```python
from build123d import *

# Parameters (mm, degrees)
F0_W     = 4
F0_H     = 1
F1_DEPTH = 1
F2_DEPTH = 6
F3_DEPTH = 2
F3_TAPER = -1


with BuildPart() as f1:
    # F0 (on Top) → F1 (new body)
    with BuildSketch(Plane.XY):
        with BuildLine():
            Line((-13, 24.5), (-12, 24.5))
            Line((-12, 24.5), (-10.5, 24.5))
            Line((-10.5, 24.5), (-8, 24.5))
            Line((-8, 24.5), (-8, 25.5))
            Line((-8, 25.5), (-8, 26.5))
            Line((-8, 26.5), (-14, 26.5))
            ThreePointArc((-14, 26.5), (-14.7071067812, 26.2071067812), (-15, 25.5))
            Line((-15, 25.5), (-15, -25.5))
            ThreePointArc((-15, -25.5), (-14.7071067812, -26.2071067812), (-14, -26.5))
            Line((-14, -26.5), (14, -26.5))
            ThreePointArc((14, -26.5), (14.7071067812, -26.2071067812), (15, -25.5))
            Line((15, -25.5), (15, 25.5))
            ThreePointArc((15, 25.5), (14.7071067812, 26.2071067812), (14, 26.5))
            Line((14, 26.5), (8, 26.5))
            Line((8, 26.5), (8, 25.5))
            Line((8, 25.5), (8, 24.5))
            Line((8, 24.5), (10.5, 24.5))
            Line((10.5, 24.5), (12, 24.5))
            ThreePointArc((12, 24.5), (12.7071067812, 24.2071067812), (13, 23.5))
            Line((13, 23.5), (13, 22))
            Line((13, 22), (13, -22))
            Line((13, -22), (13, -23.5))
            ThreePointArc((13, -23.5), (12.7071067812, -24.2071067812), (12, -24.5))
            Line((12, -24.5), (10.5, -24.5))
            Line((10.5, -24.5), (-10.5, -24.5))
            Line((-10.5, -24.5), (-12, -24.5))
            ThreePointArc((-12, -24.5), (-12.7071067812, -24.2071067812), (-13, -23.5))
            Line((-13, -23.5), (-13, -22))
            Line((-13, -22), (-13, 22))
            Line((-13, 22), (-13, 23.5))
            Line((-13, 23.5), (-13, 24.5))
        make_face()
        with Locations((6, 25)):
            Rectangle(F0_W, F0_H)
        with Locations((2, 25)):
            Rectangle(F0_W, F0_H)
        with Locations((-2, 25)):
            Rectangle(F0_W, F0_H)
        with Locations((-6, 25)):
            Rectangle(F0_W, F0_H)
        Polygon((0, 24.5), (-4, 24.5), (-4, 20), (4, 20), (4, 24.5), align=None)
        with BuildLine():
            Line((-12, -22), (-13, -22))
            Line((-13, -22), (-13, -23.5))
            ThreePointArc((-13, -23.5), (-12.7071067812, -24.2071067812), (-12, -24.5))
            Line((-12, -24.5), (-10.5, -24.5))
            Line((-10.5, -24.5), (-10.5, -23.5))
            ThreePointArc((-10.5, -23.5), (-11.5606601718, -23.0606601718), (-12, -22))
        make_face()
        with BuildLine():
            Line((-8, 24.5), (-10.5, 24.5))
            Line((-10.5, 24.5), (-10.5, 23.5))
            ThreePointArc((-10.5, 23.5), (-9.4393398282, 23.0606601718), (-9, 22))
            ThreePointArc((-9, 22), (-10.5, 20.5), (-12, 22))
            Line((-12, 22), (-13, 22))
            Line((-13, 22), (-13, -22))
            Line((-13, -22), (-12, -22))
            ThreePointArc((-12, -22), (-10.5, -20.5), (-9, -22))
            ThreePointArc((-9, -22), (-9.4393398282, -23.0606601718), (-10.5, -23.5))
            Line((-10.5, -23.5), (-10.5, -24.5))
            Line((-10.5, -24.5), (10.5, -24.5))
            Line((10.5, -24.5), (10.5, -23.5))
            ThreePointArc((10.5, -23.5), (9.4393398282, -20.9393398282), (12, -22))
            Line((12, -22), (13, -22))
            Line((13, -22), (13, 22))
            Line((13, 22), (12, 22))
            ThreePointArc((12, 22), (9.4393398282, 20.9393398282), (10.5, 23.5))
            Line((10.5, 23.5), (10.5, 24.5))
            Line((10.5, 24.5), (8, 24.5))
            Line((8, 24.5), (4, 24.5))
            Line((4, 24.5), (4, 20))
            Line((4, 20), (-4, 20))
            Line((-4, 20), (-4, 24.5))
            Line((-4, 24.5), (-8, 24.5))
        make_face()
        with BuildLine():
            Line((10.5, -23.5), (10.5, -24.5))
            Line((10.5, -24.5), (12, -24.5))
            ThreePointArc((12, -24.5), (12.7071067812, -24.2071067812), (13, -23.5))
            Line((13, -23.5), (13, -22))
            Line((13, -22), (12, -22))
            ThreePointArc((12, -22), (11.5606601718, -23.0606601718), (10.5, -23.5))
        make_face()
        with BuildLine():
            Line((12, 24.5), (10.5, 24.5))
            Line((10.5, 24.5), (10.5, 23.5))
            ThreePointArc((10.5, 23.5), (11.5606601718, 23.0606601718), (12, 22))
            Line((12, 22), (13, 22))
            Line((13, 22), (13, 23.5))
            ThreePointArc((13, 23.5), (12.7071067812, 24.2071067812), (12, 24.5))
        make_face()
        with BuildLine():
            Line((-10.5, 24.5), (-12, 24.5))
            ThreePointArc((-12, 24.5), (-12.7071067812, 24.2071067812), (-13, 23.5))
            Line((-13, 23.5), (-13, 22))
            Line((-13, 22), (-12, 22))
            ThreePointArc((-12, 22), (-11.5606601718, 23.0606601718), (-10.5, 23.5))
            Line((-10.5, 23.5), (-10.5, 24.5))
        make_face()
        with BuildLine():
            ThreePointArc((-13, 23.5), (-12.7071067812, 24.2071067812), (-12, 24.5))
            Line((-12, 24.5), (-13, 24.5))
            Line((-13, 24.5), (-13, 23.5))
        make_face()
    extrude(amount=F1_DEPTH)

    # F0 (on Top) → F2 (join)
    with BuildSketch(Plane.XY):
        with BuildLine():
            Line((-13, 24.5), (-12, 24.5))
            Line((-12, 24.5), (-10.5, 24.5))
            Line((-10.5, 24.5), (-8, 24.5))
            Line((-8, 24.5), (-8, 25.5))
            Line((-8, 25.5), (-8, 26.5))
            Line((-8, 26.5), (-14, 26.5))
            ThreePointArc((-14, 26.5), (-14.7071067812, 26.2071067812), (-15, 25.5))
            Line((-15, 25.5), (-15, -25.5))
            ThreePointArc((-15, -25.5), (-14.7071067812, -26.2071067812), (-14, -26.5))
            Line((-14, -26.5), (14, -26.5))
            ThreePointArc((14, -26.5), (14.7071067812, -26.2071067812), (15, -25.5))
            Line((15, -25.5), (15, 25.5))
            ThreePointArc((15, 25.5), (14.7071067812, 26.2071067812), (14, 26.5))
            Line((14, 26.5), (8, 26.5))
            Line((8, 26.5), (8, 25.5))
            Line((8, 25.5), (8, 24.5))
            Line((8, 24.5), (10.5, 24.5))
            Line((10.5, 24.5), (12, 24.5))
            ThreePointArc((12, 24.5), (12.7071067812, 24.2071067812), (13, 23.5))
            Line((13, 23.5), (13, 22))
            Line((13, 22), (13, -22))
            Line((13, -22), (13, -23.5))
            ThreePointArc((13, -23.5), (12.7071067812, -24.2071067812), (12, -24.5))
            Line((12, -24.5), (10.5, -24.5))
            Line((10.5, -24.5), (-10.5, -24.5))
            Line((-10.5, -24.5), (-12, -24.5))
            ThreePointArc((-12, -24.5), (-12.7071067812, -24.2071067812), (-13, -23.5))
            Line((-13, -23.5), (-13, -22))
            Line((-13, -22), (-13, 22))
            Line((-13, 22), (-13, 23.5))
            Line((-13, 23.5), (-13, 24.5))
        make_face()
        with Locations((6, 25)):
            Rectangle(F0_W, F0_H)
        with Locations((-6, 25)):
            Rectangle(F0_W, F0_H)
    extrude(amount=F2_DEPTH)

    # F0 (on Top) → F3 (join)
    with BuildSketch(Plane.XY):
        Polygon((0, 24.5), (-4, 24.5), (-4, 20), (4, 20), (4, 24.5), align=None)
    extrude(amount=F3_DEPTH, taper=F3_TAPER)


solid = f1.part
```
The model under review builds one solid part; all positions refer to its coordinate system, in mm. A direction names the side the tool comes from. Coordinates: 2 decimals unless noted, no trailing zeros. Order: outer loops, then holes, each group sorted by start corner. A loop starts at its lowest first (then second) coordinate and runs counter-clockwise, first axis right, second up. Notation, with made-up numbers: M -1,-7 L 41,-7 A14 cw 41,17 Z; hole C 4.25,61.25 d4. An arc over 180 degrees is marked long. One line per question, with ' | ' between items.
(1) For probe 1 along Y at (x, z) = (10.5, 0.55); probe 2 along X at (y, z) = (-22, 0.2); probe 3 along Y at (x, z) = (10.5, 3.5), list the stretches that pass through material, from the lowest coordinate up. Write a range as from..to.
Geometry results:
probe 1: y = -26.5..-23.5, -20.5..20.5, 23.5..26.5 | probe 2: x = -15..-12, -9..9, 12..15 | probe 3: y = -26.5..-24.5, 24.5..26.5
(2) The part is to be moulded in two halves that separate along Y. For faces 1 (the face through (-1, 0, 0)), 2 (the face through (0, 0, 1)), 3 (the face through (-14.699, 26.215, 2.958)), 4 (the face through (-13, 0, 3)), say which applies: +Y half, -Y half, draft (parallel to the pull), parting line (faces both ways), or undercut.
Geometry results:
face 1: draft | face 2: undercut | face 3: +Y half | face 4: undercut
(3) Machinability: for faces 5 (the face through (14.715, 26.199, 2.958)), 6 (the face through (0.1, 25.5, 0.3)), 7 (the face through (12.699, 24.215, 3.465)), which of the approach directions +Z, -Z, +X, -X, +Y, -Y give a long, thin tool a straight path to every point of the face, cutting with its end or side? Answer none if there is none.
Geometry results:
face 5: +Z, -Z, +X, +Y | face 6: +Z, -Z, +Y | face 7: +Z
(4) Insertion check: pin 1 (13 mm diameter, centred on x = 2.5, y = 7.5, fed in from +Z); pin 2 (1.4 mm diameter, centred on x = -1, y = 22, fed in from +Z); pin 3 (1.5 mm diameter, centred on x = -1, z = 2.5, fed in from +Y). Each pin has a flat end and moves straight along its axis. Give the tip position at first contact, or say it passes through.
Geometry results:
pin 1: stops at z = 1 | pin 2: stops at z = 2 | pin 3: stops at y = 24.53
(5) Add section C-C, the plane z = 4.5. Write out the cut boundary in (x, y).
Geometry results:
outline: M -15,-25.5 A1 ccw -14,-26.5 L 14,-26.5 A1 ccw 15,-25.5 L 15,25.5 A1 ccw 14,26.5 L 8,26.5 L 8,25.5 L 4,25.5 L 4,24.5 L 12,24.5 A1 cw 13,23.5 L 13,-23.5 A1 cw 12,-24.5 L -12,-24.5 A1 cw -13,-23.5 L -13,24.5 L -4,24.5 L -4,25.5 L -8,25.5 L -8,26.5 L -14,26.5 A1 ccw -15,25.5 Z
(6) Add section B-B, the plane y = -21. Write out the cut boundary in (x, z), then the cut area to 3 significant figures.
Geometry results:
outline: M -15,0 L -11.62,0 L -11.62,1 L -13,1 L -13,6 L -15,6 Z; M -9.38,0 L 9.38,0 L 9.38,1 L -9.38,1 Z; M 11.62,0 L 15,0 L 15,6 L 13,6 L 13,1 L 11.62,1 Z | area: 45.5 mm²
(7) Add section D-D, the plane y = -7. Write out the cut boundary in (x, z).
Geometry results:
outline: M -15,0 L 15,0 L 15,6 L 13,6 L 13,1 L -13,1 L -13,6 L -15,6 Z
(8) Add section A-A, the plane x = -8.5. Write out the cut boundary in (y, z).
Geometry results:
outline: M -26.5,0 L 26.5,0 L 26.5,6 L 24.5,6 L 24.5,1 L -24.5,1 L -24.5,6 L -26.5,6 Z
